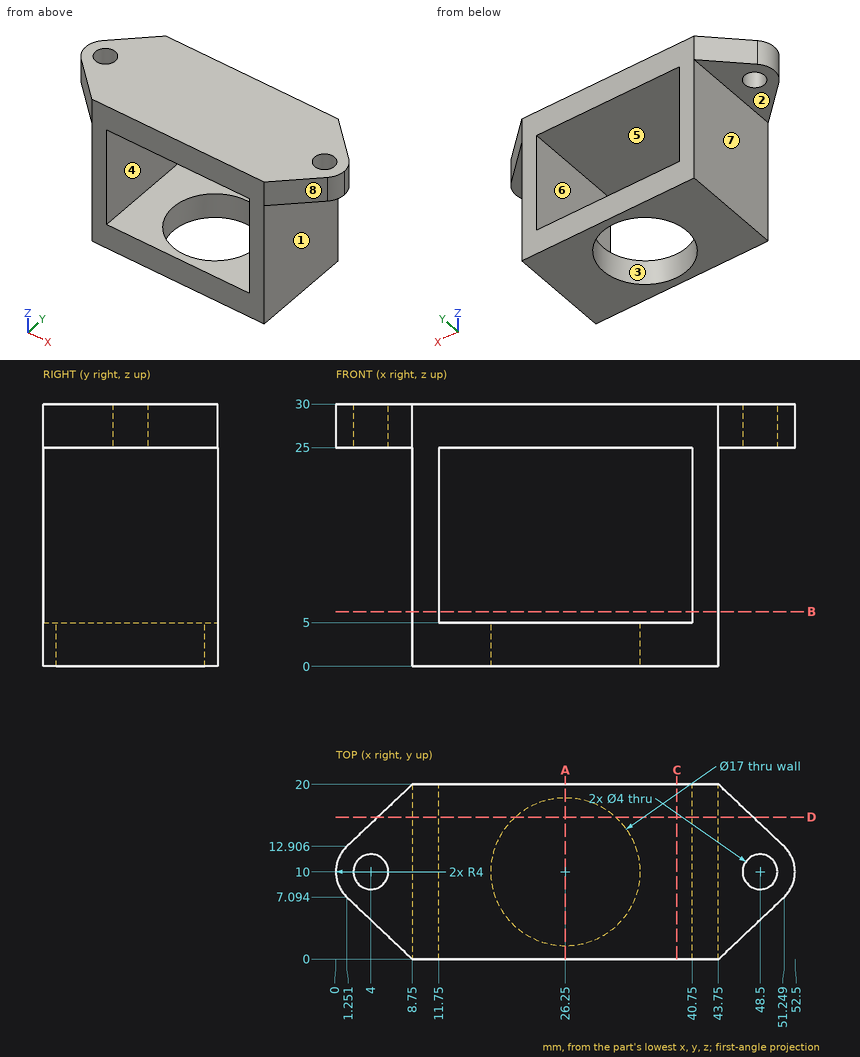
Can you work these out from the drawing? Everything is in mm from the part's minimum corner. A direction names the side the tool comes from. Round coordinates to 2 decimals unless told otherwise and drop trailing zeros. Loops run counter-clockwise (first coordinate to the right, second up) from the corner with the lowest first, then second, coordinate; pieces in that order, holes last.
1. If I drill on line 1 along X through (y, z) = (11.5, 22.5); line 2 along Z through (x, y) = (36, 15); line 3 along Y through (x, z) = (26.25, 2), over which ranges is the centre line in solid material (lowest first)?
Answer list:
line 1: x = 8.75 to 11.75, 40.75 to 43.75
line 2: z = 0 to 5, 25 to 30
line 3: y = 0 to 1.5, 18.5 to 20
2. If we section it at B-B on z = 6.25: Write out the boundary of the cut face in (x, y).
Answer list:
outline: (8.75, 0) - (11.75, 0) - (11.75, 20) - (8.75, 20) - close; (40.75, 0) - (43.75, 0) - (43.75, 20) - (40.75, 20) - close
3. If we section it at A-A on x = 26.25: Write out the boundary of the cut face in (y, z).
Answer list:
outline: (0, 0) - (1.5, 0) - (1.5, 5) - (0, 5) - close; (0, 25) - (20, 25) - (20, 30) - (0, 30) - close; (18.5, 0) - (20, 0) - (20, 5) - (18.5, 5) - close
4. We'd pull the mould along X, two halves only. Please class the marked faces 5, 6, 7 and 8: +X half, -X half, draft (parallel to the pull), parting line (faces both ways), or undercut.
Answer list:
face 5: undercut
face 6: undercut
face 7: -X half
face 8: +X half
5. If we section it at D-D on y = 16.25: Write out the boundary of the cut face in (x, z), plus the area to 3 significant figures.
Answer list:
outline: (4.79, 25) - (8.75, 25) - (8.75, 0) - (20.49, 0) - (20.49, 5) - (11.75, 5) - (11.75, 25) - (40.75, 25) - (40.75, 5) - (32.01, 5) - (32.01, 0) - (43.75, 0) - (43.75, 25) - (47.71, 25) - (47.71, 30) - (4.79, 30) - close
area: 452 mm2
6. Which directions (+Z, -Z, +X, -X, +Y, -Y) give clear straight access to the entire face, cutting with the end or side of a thin tool? Please do the marked faces 1, 2, 3 and 4.
Answer list:
face 1: -Z, +X, +Y, -Y
face 2: -Z, -X, +Y, -Y
face 3: -Z
face 4: +Y, -Y
7. If we section it at C-C on x = 39: Write out the boundary of the cut face in (y, z), plus the area to 3 significant figures.
Answer list:
outline: (0, 0) - (20, 0) - (20, 5) - (0, 5) - close; (0, 25) - (20, 25) - (20, 30) - (0, 30) - close
area: 200 mm2
8. For P1, Ø7, axis at x = 48.5, y = 11.5, coming from the -Z side; P2, Ø10, axis at y = 14.5, z = 12.5, coming from the +X side; P3, Ø6, axis at y = 17.5, z = 10, coming from the -X side, each with a flat end and sliding along its axis, tell me the tip position at first contact or that it passes through.
Answer list:
P1: stops at z = 25
P2: stops at x = 43.75
P3: stops at x = 8.75
